Work out the finished part from the listing and answer in its coordinate system (mm). Face numbers are marked on the shaded views. A direction names the side the tool comes from. Round coordinates to 2 decimals unless told otherwise and drop trailing zeros. Loops run counter-clockwise (first coordinate to the right, second up) from the corner with the lowest first, then second, coordinate; pieces in that order, holes last. Notation, with made-up numbers: M 3,35 L 10,35 A27 cw 10,54 Z; hole C -33,73 d7. An arc over 180 degrees is marked long. One line per item, written item: value.
```python
from build123d import *

# Parameters (mm, degrees)
BOSS_EXTRUDE1_DEPTH = 60
SKETCH1_4_R         = 6.338999997
SKETCH1_4_R_2       = 3.302
SKETCH1_4_R_3       = 3.301999997
BOSS_EXTRUDE2_DEPTH = 10
SKETCH1_6_R         = 6.338999997
SKETCH1_6_R_2       = 3.301999997
SKETCH1_6_R_3       = 3.302
BOSS_EXTRUDE4_DEPTH = 30
BOSS_EXTRUDE5_DEPTH = 60
BOSS_EXTRUDE6_START = -2
BOSS_EXTRUDE6_DEPTH = 6
CIRPATTERN3_COUNT   = 16


# Read off the part's stored shape, not the designer's step: Boss-Extrude1
with BuildPart() as part:
    # Boss-Extrude1 outline → Boss-Extrude1 (new body)
    with BuildSketch(Plane.XY):
        with BuildLine():
            Line((-27.424137764, 42.49999995), (-15.877132386, 22.499999959))
            Line((-15.877132386, 22.499999959), (-22.542678391, 10.954935617))
            ThreePointArc((-22.542678391, 10.954935617), (-32.536728065, -0.49784941), (-21.547999925, -11.00000003))
            Line((-21.547999925, -11.00000003), (-10.999999983, -11.00000003))
            Line((-10.999999983, -11.00000003), (-10.999999983, -21.547999949))
            ThreePointArc((-10.999999983, -21.547999949), (2.4e-08, -32.547999956), (11.00000003, -21.547999949))
            Line((11.00000003, -21.547999949), (11.00000003, -11.000000006))
            Line((11.00000003, -11.000000006), (21.547999949, -11.000000006))
            ThreePointArc((21.547999949, -11.000000006), (32.53672809, -0.497849376), (22.542678394, 10.954935643))
            Line((22.542678394, 10.954935643), (15.877132386, 22.499999959))
            Line((15.877132386, 22.499999959), (27.424137764, 42.49999995))
            Line((27.424137764, 42.49999995), (53.404899911, 42.49999995))
            Line((53.404899911, 42.49999995), (66.39528096, 64.999999935))
            Line((66.39528096, 64.999999935), (69.282032276, 65.000000028))
            ThreePointArc((69.282032276, 65.000000028), (63.510032668, 70.650376861), (57.278911905, 75.79001419))
            Line((57.278911905, 75.79001419), (62.0651539, 67.499999879))
            Line((62.0651539, 67.499999879), (50.518148521, 47.499999888))
            Line((50.518148521, 47.499999888), (27.42413776, 47.499999896))
            Line((27.42413776, 47.499999896), (15.877132386, 67.499999879))
            Line((15.877132386, 67.499999879), (27.424137764, 87.49999987))
            Line((27.424137764, 87.49999987), (36.996621947, 87.499999797))
            ThreePointArc((36.996621947, 87.499999797), (29.430004911, 90.326490085), (21.650635056, 92.500000009))
            Line((21.650635056, 92.500000009), (23.094010837, 89.999999729))
            Line((23.094010837, 89.999999729), (11.547005507, 69.999999822))
            Line((11.547005507, 69.999999822), (-11.547004687, 69.999999822))
            Line((-11.547004687, 69.999999822), (-23.094010614, 89.999999911))
            Line((-23.094010614, 89.999999911), (-21.650634856, 92.500000056))
            ThreePointArc((-21.650634856, 92.500000056), (-29.430004813, 90.326490116), (-36.996621947, 87.499999797))
            Line((-36.996621947, 87.499999797), (-27.424137764, 87.49999987))
            Line((-27.424137764, 87.49999987), (-15.877132386, 67.499999879))
            Line((-15.877132386, 67.499999879), (-27.424137764, 47.499999888))
            Line((-27.424137764, 47.499999888), (-50.518148521, 47.499999888))
            Line((-50.518148521, 47.499999888), (-62.0651539, 67.499999879))
            Line((-62.0651539, 67.499999879), (-57.278911905, 75.79001419))
            ThreePointArc((-57.278911905, 75.79001419), (-63.510032668, 70.650376861), (-69.282032276, 65.000000028))
            Line((-69.282032276, 65.000000028), (-66.39528096, 64.999999935))
            Line((-66.39528096, 64.999999935), (-53.404899911, 42.49999995))
            Line((-53.404899911, 42.49999995), (-27.424137764, 42.49999995))
        make_face()
        Polygon((-11.000000006, 19.999999941), (-11.000000006, 10.999999983), (-16.743157748, 10.999999983), (-11.54700535, 19.999999941), align=None, mode=Mode.SUBTRACT)
        with BuildLine():
            Line((-9.767988869, -5.058299477), (-17.727459778, -5.058299515))
            ThreePointArc((-17.727459778, -5.058299515), (-27.88699994, -4.1e-08), (-17.727459815, 5.058299508))
            Line((-17.727459815, 5.058299508), (-9.767988835, 5.058299543))
            ThreePointArc((-9.767988835, 5.058299543), (-7.778174571, 7.778174624), (-5.058299477, 9.767988869))
            Line((-5.058299477, 9.767988869), (-5.058299513, 17.727459781))
            ThreePointArc((-5.058299513, 17.727459781), (-1.2e-08, 27.886999922), (5.058299528, 17.7274598))
            Line((5.058299528, 17.7274598), (5.058299543, 9.767988835))
            ThreePointArc((5.058299543, 9.767988835), (7.778174624, 7.778174571), (9.767988869, 5.058299477))
            Line((9.767988869, 5.058299477), (17.727459795, 5.058299493))
            ThreePointArc((17.727459795, 5.058299493), (27.88699994, -1.5e-08), (17.727459798, -5.05829953))
            Line((17.727459798, -5.05829953), (9.767988835, -5.058299543))
            ThreePointArc((9.767988835, -5.058299543), (7.778174571, -7.778174624), (5.058299477, -9.767988869))
            Line((5.058299477, -9.767988869), (5.058299496, -17.727459793))
            ThreePointArc((5.058299496, -17.727459793), (1.3e-08, -27.886999957), (-5.058299511, -17.727459813))
            Line((-5.058299511, -17.727459813), (-5.058299543, -9.767988835))
            ThreePointArc((-5.058299543, -9.767988835), (-7.778174624, -7.778174571), (-9.767988869, -5.058299477))
        make_face(mode=Mode.SUBTRACT)
        Polygon((16.743157694, 11.000000006), (11.000000006, 11.000000006), (11.000000006, 19.999999941), (11.54700535, 19.999999941), align=None, mode=Mode.SUBTRACT)
        with BuildLine():
            Line((23.094010708, 44.999999885), (11.547005356, 24.999999941))
            Line((11.547005356, 24.999999941), (10.444314053, 24.999999941))
            ThreePointArc((10.444314053, 24.999999941), (0, 32.547999932), (-10.444314053, 24.999999941))
            Line((-10.444314053, 24.999999941), (-11.547005099, 24.999999941))
            Line((-11.547005099, 24.999999941), (-23.094010665, 44.999999941))
            Line((-23.094010665, 44.999999941), (-11.54700535, 64.999999822))
            Line((-11.54700535, 64.999999822), (11.54700535, 64.999999822))
            Line((11.54700535, 64.999999822), (23.094010708, 44.999999885))
        make_face(mode=Mode.SUBTRACT)
    extrude(amount=BOSS_EXTRUDE1_DEPTH)

    # Sketch1<4> → Boss-Extrude2 (add)
    # profile 1 of 4: a face of its own
    with BuildSketch(Plane.XY):
        with Locations((0, 21.547999925)):
            Circle(SKETCH1_4_R)
        with Locations((0, 21.547999925)):
            Circle(SKETCH1_4_R_2, mode=Mode.SUBTRACT)
    # profile 2 of 4: a face of its own
    with BuildSketch(Plane.XY):
        with Locations((21.547999943, -1.7e-08)):
            Circle(SKETCH1_4_R)
        with Locations((21.547999974, -2.6e-08)):
            Circle(SKETCH1_4_R_2, mode=Mode.SUBTRACT)
    # profile 3 of 4: a face of its own
    with BuildSketch(Plane.XY):
        with Locations((-21.547999943, -1.7e-08)):
            Circle(SKETCH1_4_R)
        with Locations((-21.547999951, -4.8e-08)):
            Circle(SKETCH1_4_R_2, mode=Mode.SUBTRACT)
    # profile 4 of 4: a face of its own
    with BuildSketch(Plane.XY):
        with Locations((0, -21.54799996)):
            Circle(SKETCH1_4_R)
        with Locations((2.3e-08, -21.547999999)):
            Circle(SKETCH1_4_R_3, mode=Mode.SUBTRACT)
    extrude(amount=BOSS_EXTRUDE2_DEPTH)

    # Sketch1<6> → Boss-Extrude4 (add)
    # profile 1 of 4: a face of its own
    with BuildSketch(Plane.XY):
        with Locations((0, -21.54799996)):
            Circle(SKETCH1_6_R)
        with Locations((2.3e-08, -21.547999999)):
            Circle(SKETCH1_6_R_2, mode=Mode.SUBTRACT)
    # profile 2 of 4: a face of its own
    with BuildSketch(Plane.XY):
        with Locations((-21.547999943, -1.7e-08)):
            Circle(SKETCH1_6_R)
        with Locations((-21.547999951, -4.8e-08)):
            Circle(SKETCH1_6_R_3, mode=Mode.SUBTRACT)
    # profile 3 of 4: a face of its own
    with BuildSketch(Plane.XY):
        with Locations((21.547999943, -1.7e-08)):
            Circle(SKETCH1_6_R)
        with Locations((21.547999974, -2.6e-08)):
            Circle(SKETCH1_6_R_3, mode=Mode.SUBTRACT)
    # profile 4 of 4: a face of its own
    with BuildSketch(Plane.XY):
        with Locations((0, 21.547999925)):
            Circle(SKETCH1_6_R)
        with Locations((0, 21.547999925)):
            Circle(SKETCH1_6_R_3, mode=Mode.SUBTRACT)
    extrude(amount=BOSS_EXTRUDE4_DEPTH)

    # Sketch1<7> → Boss-Extrude5 (add)
    with BuildSketch(Plane.XY):
        with BuildLine():
            Line((-69.282032276, 65.000000028), (-72.928455025, 68.421052659))
            ThreePointArc((-72.928455025, 68.421052659), (0, 99.999999996), (72.928455025, 68.421052659))
            Line((72.928455025, 68.421052659), (69.282032276, 65.000000028))
            ThreePointArc((69.282032276, 65.000000028), (0, 95), (-69.282032276, 65.000000028))
        make_face()
    extrude(amount=BOSS_EXTRUDE5_DEPTH)

    # Sketch2 → Boss-Extrude6 (add)
    with BuildSketch(Plane(origin=(49.999999998, 86.602540375, 0), x_dir=(0.866025403784439, -0.4999999999999993, 0), z_dir=(0.4999999999999993, 0.866025403784439, 0)).offset(BOSS_EXTRUDE6_START)):
        with BuildLine():
            Line((0, 0), (-5, 0))
            add(Edge.make_bspline(
                [(-5, 0), (4.762549661, -30.076815137), (-5.473720523, -60)],
                knots=[0, 0, 0, 1, 1, 1], degree=2))
            Line((-5.473720523, -60), (-0.473720523, -60))
            add(Edge.make_bspline(
                [(0, 0), (9.762549647, -30.076815137), (-0.473720523, -60)],
                knots=[0, 0, 0, 1, 1, 1], degree=2))
        make_face()
    boss_extrude6 = extrude(amount=BOSS_EXTRUDE6_DEPTH)

    # CirPattern3: Boss-Extrude6 ×16 about axis, 12 skipped
    cirpattern3_axis = Axis((0, 0, 0), (0, 0, -1))
    add([boss_extrude6.rotate(cirpattern3_axis, i * 360 / CIRPATTERN3_COUNT) for i in range(1, CIRPATTERN3_COUNT) if i not in (1, 2, 3, 4, 5, 6, 7, 8, 9, 10, 11, 12)])


solid = part.part
```
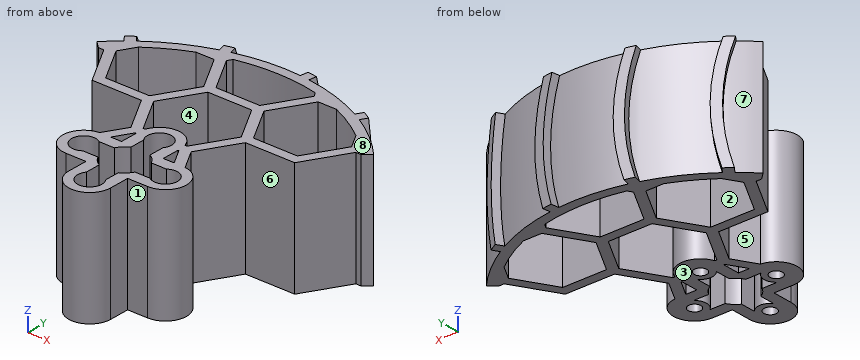
1) Each of these flat-tipped pins is pushed along its axis until it touches: pin 1 (3 mm diameter, centred on y = 29, z = 12, fed in from +X); pin 2 (8 mm diameter, centred on x = -51, z = 21, fed in from -Y); pin 3 (3 mm diameter, centred on y = -14, z = 20, fed in from +X). Where does it stop, or does it pass through?
Check values:
pin 1: x = 20.5
pin 2: y = 42.5
pin 3: x = 11
2) Find section B-B (y = 61.5). Give the vertices of the cut face in (x, z), then the cut area to 3 significant figures.
Check values:
outline: M -64.37,0 L -58.6,0 L -58.6,60 L -64.37,60 Z; M -19.34,0 L -13.57,0 L -13.57,60 L -19.34,60 Z; M 13.57,0 L 19.34,0 L 19.34,60 L 13.57,60 Z; M 58.6,0 L 64.37,0 L 64.37,60 L 58.6,60 Z
area: 1,390 mm2
3) For the marked faces 4, 5, 6, 7 and 8, determine the directions among +Z, -Z, +X, -X, +Y, -Y from which every point of the face is accessible in a straight line to the end or side of a thin tool.
Check values:
face 4: +Z, -Z
face 5: +Z, -Z, -X
face 6: +Z, -Z, +X
face 7: -X
face 8: +Z, +X, -X, +Y, -Y
4) The mould has two halves that part along Y. Classify the marked faces 1, 2 and 3: +Y half, -Y half, draft (parallel to the pull), parting line (faces both ways), or undercut.
Check values:
face 1: -Y half
face 2: undercut
face 3: draft
5) Find section C-C (y = 0). Give the vertices of the cut face in (x, z).
Check values:
outline: M -32.55,0 L -24.85,0 L -24.85,30 L -27.89,30 L -27.89,60 L -32.55,60 Z; M -18.25,0 L -15.21,0 L -15.21,30 L -18.25,30 Z; M 15.21,0 L 18.25,0 L 18.25,30 L 15.21,30 Z; M 24.85,0 L 32.55,0 L 32.55,60 L 27.89,60 L 27.89,30 L 24.85,30 Z
6) Find the intervals of material crossed by probe 1 along X at (y, z) = (-15, 17.5); probe 2 along Y at (x, z) = (-18, 23.5); probe 3 along X at (y, z) = (3, 10), in increasing order. Write a range as from..to.
Check values:
probe 1: -11..-5.06, 5.06..11
probe 2: -11..18.82, 26.18..36.18, 53.82..63.82, 71.18..81.18, 93.28..98.37
probe 3: -32.13..-22.93, -20.17..-15.96, 15.96..20.17, 22.93..32.13
7) Find section D-D (z = 50.5). Give the number of separate pieces and of enclosed holes in the cut face, then the cut area to 3 significant figures.
Check values:
separate pieces: 1
enclosed holes: 7
area: 3,560 mm2
8) Find section A-A (x = 0). Give the vertices of the cut face in (y, z), then the cut area to 3 significant figures.
Check values:
outline: M -32.55,0 L -24.85,0 L -24.85,30 L -27.89,30 L -27.89,60 L -32.55,60 Z; M -18.25,0 L -15.21,0 L -15.21,30 L -18.25,30 Z; M 15.21,0 L 18.25,0 L 18.25,30 L 15.21,30 Z; M 24.85,0 L 32.55,0 L 32.55,60 L 27.89,60 L 27.89,30 L 24.85,30 Z; M 65,0 L 70,0 L 70,60 L 65,60 Z; M 95,0 L 100,0 L 100,60 L 95,60 Z
area: 1,520 mm2
